```python
from build123d import *

# Parameters (mm, degrees)
SKETCH1_R           = 2.25
SKETCH1_R_2         = 1.65
BOSS_EXTRUDE1_DEPTH = 2
BOSS_EXTRUDE2_DEPTH = 5


with BuildPart() as part:
    # Sketch1 → Boss-Extrude1 (new body)
    with BuildSketch(Plane.XY):
        with BuildLine():
            Line((-4.14, -8.9), (-3.94, -8.9))
            Line((-3.94, -8.9), (-3.94, -5.942048338))
            ThreePointArc((-3.94, -5.942048338), (-6.111467123, -4.707426407), (-7.919595949, -2.983990617))
            Line((-7.919595949, -2.983990617), (-11.186429278, 0.282842712))
            ThreePointArc((-11.186429278, 0.282842712), (-11.245007922, 0.424264069), (-11.186429278, 0.565685425))
            Line((-11.186429278, 0.565685425), (-0.565685425, 11.186429278))
            ThreePointArc((-0.565685425, 11.186429278), (-0.424264069, 11.245007922), (-0.282842712, 11.186429278))
            Line((-0.282842712, 11.186429278), (2.983990617, 7.919595949))
            ThreePointArc((2.983990617, 7.919595949), (5.746266235, 4.38042767), (6.73, 0))
            ThreePointArc((6.73, 0), (5.992040554, -3.064041449), (3.94, -5.456124999))
            Line((3.94, -5.456124999), (3.94, -8.9))
            Line((3.94, -8.9), (4.14, -8.9))
            ThreePointArc((4.14, -8.9), (5.44, -10.2), (4.14, -11.5))
            Line((4.14, -11.5), (3.94, -11.5))
            Line((3.94, -11.5), (3.94, -12.8))
            ThreePointArc((3.94, -12.8), (3.852132034, -13.012132034), (3.64, -13.1))
            Line((3.64, -13.1), (-3.64, -13.1))
            ThreePointArc((-3.64, -13.1), (-3.852132034, -13.012132034), (-3.94, -12.8))
            Line((-3.94, -12.8), (-3.94, -11.5))
            Line((-3.94, -11.5), (-4.14, -11.5))
            ThreePointArc((-4.14, -11.5), (-5.44, -10.2), (-4.14, -8.9))
        make_face()
        Circle(SKETCH1_R, mode=Mode.SUBTRACT)
        with Locations((0, -10.2)):
            Circle(SKETCH1_R_2, mode=Mode.SUBTRACT)
    extrude(amount=BOSS_EXTRUDE1_DEPTH)

    # Sketch2 → Boss-Extrude2 (add)
    with BuildSketch(Plane.XY.offset(2)):
        with BuildLine():
            Line((0.700035713, 6.781154032), (1.272792206, 6.208397539))
            ThreePointArc((1.272792206, 6.208397539), (1.414213562, 6.149818895), (1.555634919, 6.208397539))
            Line((1.555634919, 6.208397539), (2.983990617, 7.636753237))
            ThreePointArc((2.983990617, 7.636753237), (3.04256926, 7.778174593), (2.983990617, 7.919595949))
            Line((2.983990617, 7.919595949), (-0.282842712, 11.186429278))
            ThreePointArc((-0.282842712, 11.186429278), (-0.424264069, 11.245007922), (-0.565685425, 11.186429278))
            Line((-0.565685425, 11.186429278), (-11.186429278, 0.565685425))
            ThreePointArc((-11.186429278, 0.565685425), (-11.245007922, 0.424264069), (-11.186429278, 0.282842712))
            Line((-11.186429278, 0.282842712), (-7.919595949, -2.983990617))
            ThreePointArc((-7.919595949, -2.983990617), (-7.778174593, -3.04256926), (-7.636753237, -2.983990617))
            Line((-7.636753237, -2.983990617), (-6.208397539, -1.555634919))
            ThreePointArc((-6.208397539, -1.555634919), (-6.149818895, -1.414213562), (-6.208397539, -1.272792206))
            Line((-6.208397539, -1.272792206), (-6.781154032, -0.700035713))
            ThreePointArc((-6.781154032, -0.700035713), (-6.922575388, -0.64145707), (-7.063996744, -0.700035713))
            Line((-7.063996744, -0.700035713), (-7.636753237, -1.272792206))
            ThreePointArc((-7.636753237, -1.272792206), (-7.778174593, -1.33137085), (-7.919595949, -1.272792206))
            Line((-7.919595949, -1.272792206), (-8.414570696, -0.777817459))
            ThreePointArc((-8.414570696, -0.777817459), (-8.47314934, -0.636396103), (-8.414570696, -0.494974747))
            Line((-8.414570696, -0.494974747), (-7.841814203, 0.077781746))
            ThreePointArc((-7.841814203, 0.077781746), (-7.78323556, 0.219203102), (-7.841814203, 0.360624458))
            Line((-7.841814203, 0.360624458), (-8.619631663, 1.138441918))
            ThreePointArc((-8.619631663, 1.138441918), (-8.678210306, 1.279863274), (-8.619631663, 1.42128463))
            Line((-8.619631663, 1.42128463), (-1.42128463, 8.619631663))
            ThreePointArc((-1.42128463, 8.619631663), (-1.279863274, 8.678210306), (-1.138441918, 8.619631663))
            Line((-1.138441918, 8.619631663), (-0.360624458, 7.841814203))
            ThreePointArc((-0.360624458, 7.841814203), (-0.219203102, 7.78323556), (-0.077781746, 7.841814203))
            Line((-0.077781746, 7.841814203), (0.494974747, 8.414570696))
            ThreePointArc((0.494974747, 8.414570696), (0.636396103, 8.47314934), (0.777817459, 8.414570696))
            Line((0.777817459, 8.414570696), (1.272792206, 7.919595949))
            ThreePointArc((1.272792206, 7.919595949), (1.33137085, 7.778174593), (1.272792206, 7.636753237))
            Line((1.272792206, 7.636753237), (0.700035713, 7.063996744))
            ThreePointArc((0.700035713, 7.063996744), (0.64145707, 6.922575388), (0.700035713, 6.781154032))
        make_face()
    extrude(amount=BOSS_EXTRUDE2_DEPTH)


solid = part.part
```
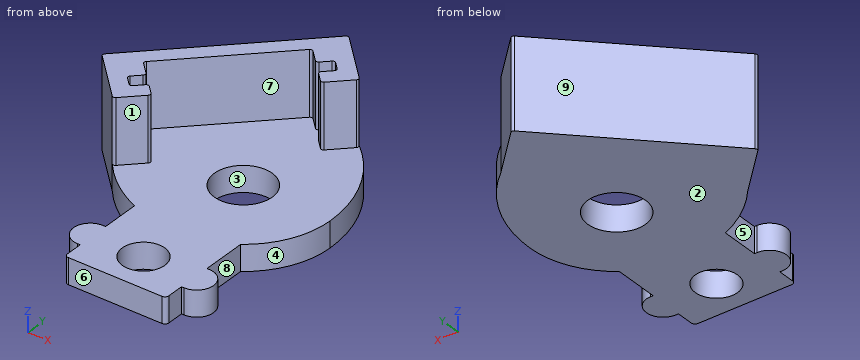
Input: part model. Units: mm. Frame: model coordinates. Face numbers are marked on the shaded views. A direction names the side the tool comes from. Round coordinates to 2 decimals unless told otherwise and drop trailing zeros. Loops run counter-clockwise (first coordinate to the right, second up) from the corner with the lowest first, then second, coordinate; pieces in that order, holes last. Notation, with made-up numbers: (-40, 32.25) - (-17, 32.25) arc R11 ccw to (-17, 37.25) - close; hole circle Ø7 at (27, 53.5). An arc over 180 degrees is marked (long way). One line per item, written item: value. Start each with the question number.
(1) Contact query for flat-ended pins moving along their axis: P1, Ø1.6, axis at y = -8, z = 1.5, coming from the -X side; P2, Ø5, axis at x = -3.5, y = -9.5, coming from the +Z side; P3, Ø1.6, axis at y = -6.5, z = 1, coming from the +X side. Output: stop coordinate, or through.
(2) Access query for the marked faces 1, 2, 3, 4 and 5. Directions: +Z, -Z, +X, -X, +Y, -Y. A direction counts if a zero-diameter tool reaches every point of the face in a straight line with its end or side. Return the directions, or none.
(3) Ray query, line 1 (Y direction, x = 0, z = 0.55); line 2 (Z direction, x = -1.25, y = -9); line 3 (X direction, y = 0.5, z = 0.5). Return the intervals inside material, ascending. Write a range as [from, to].
(4) Section C-C, the plane y = -2. Return loops of the section in (x, z).
(5) Section D-D, the plane x = 5.75. Return loops of the section in (y, z), plus the area to 3 significant figures.
(6) Draft query along Y for the marked faces 6, 7, 8 and 9. Return one class per face: +Y half, -Y half, draft (parallel to the pull), parting line (faces both ways), or undercut.
(7) Section A-A, the plane y = -10.2. Return loops of the section in (x, z), plus the area to 3 significant figures.
Results below:
1. P1: x = -3.94
1. P2: z = 2
1. P3: x = 3.94
2. face 1: +Z, +X, -Y
2. face 2: -Z, +X, -X, +Y, -Y
2. face 3: +Z, -Z
2. face 4: +Z, -Z, +X
2. face 5: +Z, -Z, -X
3. line 1: [-13.1, -11.85], [-8.55, -2.25], [2.25, 10.9]
3. line 2: [0, 2]
3. line 3: [-11.23, -2.19], [2.19, 6.72]
4. outline: (-8.9, 0) - (-1.03, 0) - (-1.03, 2) - (-6.65, 2) - (-6.65, 7) - (-8.9, 7) - close; (1.03, 0) - (6.43, 0) - (6.43, 2) - (1.03, 2) - close
5. outline: (-3.5, 0) - (4.37, 0) - (4.37, 2) - (-3.5, 2) - close
5. area: 15.7 mm^2
6. face 6: -Y half
6. face 7: undercut
6. face 8: undercut
6. face 9: +Y half
7. outline: (-5.44, 0) - (-1.65, 0) - (-1.65, 2) - (-5.44, 2) - close; (1.65, 0) - (5.44, 0) - (5.44, 2) - (1.65, 2) - close
7. area: 15.2 mm^2
